from build123d import *
from build123d.topology import SkipClean

# Parameters (mm, degrees)
BOSS_EXTRUDE1_DEPTH = 44.45
BOSS_EXTRUDE2_DEPTH = 25.4
BOSS_EXTRUDE3_START = -6.35
BOSS_EXTRUDE3_DEPTH = 6.35


with BuildPart() as part:
    # Sketch1 → Boss-Extrude1 (new body)
    with BuildSketch(Plane(origin=(0, 0, 0), x_dir=(1, 0, 0), z_dir=(0, 1, 0))):
        with BuildLine():
            Line((-3.941092361, 3), (3.941092361, 3))
            ThreePointArc((3.941092361, 3), (0, -4.953), (-3.941092361, 3))
        make_face()
    extrude(amount=BOSS_EXTRUDE1_DEPTH)

    # Sketch3 → Boss-Extrude2 (add)
    with SkipClean():  # the faces are left unmerged after this step: merging them gives an invalid solid
        with BuildSketch(Plane.XZ):
            with BuildLine():
                Line((-3.941092361, -3), (3.941092361, -3))
                ThreePointArc((3.941092361, -3), (0, -4.953), (-3.941092361, -3))
            make_face()
        extrude(amount=-BOSS_EXTRUDE2_DEPTH)

    # Sketch4 → Boss-Extrude3 (add)
    with SkipClean():  # the faces are left unmerged after this step: merging them gives an invalid solid
        with BuildSketch(Plane(origin=(0, 44.45, 0), x_dir=(1, 0, 0), z_dir=(0, 1, 0)).offset(BOSS_EXTRUDE3_START)):
            with BuildLine():
                Line((-3.941092361, 3), (3.941092361, 3))
                ThreePointArc((3.941092361, 3), (0, 4.953), (-3.941092361, 3))
            make_face()
        extrude(amount=BOSS_EXTRUDE3_DEPTH)


solid = part.part
Model file for the job. Use its own axes, mm. Give positions to 0.01 mm unless a question says otherwise; leave off trailing zeros. Loops run counter-clockwise (first coordinate to the right, second up) from the corner with the lowest first, then second, coordinate; pieces in that order, holes last.
1) Flat gauge pin, fed straight in: pin 1 Ø2.5 at (x, y) = (1, 34.5) entering from -Z. Where does the tip first touch, or does it go through?
2) Saw through at C-C (x = -2.5). Write the cut outline in (y, z).
3) Saw through at A-A (x = 0). Write the cut outline in (y, z).
4) Saw through at B-B (y = 6.5). Write the cut outline in (x, z), plus the area to 3 significant figures.
5) Wall check: line 1 (Y direction, x = -2.5, z = -3.5); line 2 (Z direction, x = 0.25, y = 20); line 3 (Z direction, x = 2, y = 27.5). Give the ranges that are in metal, low to high.
6) Pull direction Y, two halves, no side cores. Call faces 1 (the flat face through (0, 0, 0)), 2 (the flat face through (0, 44.45, 0)), 3 (the flat face through (0, 32, -3)): +Y half, -Y half, draft (parallel to the pull), parting line (faces both ways), or undercut.
7) Saw through at D-D (z = -1.5). Write the cut outline in (x, y), plus the area to 3 significant figures.
Answer block:
1. pin 1: stops at z = -3
2. outline: (0, -4.28) - (25.4, -4.28) - (25.4, -3) - (38.1, -3) - (38.1, -4.28) - (44.45, -4.28) - (44.45, 4.28) - (0, 4.28) - close
3. outline: (0, -4.95) - (25.4, -4.95) - (25.4, -3) - (38.1, -3) - (38.1, -4.95) - (44.45, -4.95) - (44.45, 4.95) - (0, 4.95) - close
4. outline: circle Ø9.91 at (0, 0)
4. area: 77.1 mm2
5. line 1: y = 0 to 25.4, 38.1 to 44.45
5. line 2: z = -4.95 to 4.95
5. line 3: z = -3 to 4.53
6. face 1: -Y half
6. face 2: +Y half
6. face 3: undercut
7. outline: (-4.72, 0) - (4.72, 0) - (4.72, 44.45) - (-4.72, 44.45) - close
7. area: 420 mm2
